The listing builds one solid part. Answer for the finished solid, in the listing's coordinates (mm). A direction names the side the tool comes from. Round coordinates to 2 decimals unless told otherwise and drop trailing zeros. Use a Markdown table: item, result. Add a question column.
Q1. Given pin 1 Ø6 at (x, y) = (-12.5, -16) entering from +Z; pin 2 Ø3 at (y, z) = (-13.5, 18) entering from +X; pin 3 Ø10 at (y, z) = (-21, -25) entering from +X, each flat-ended and moving along its own axis, determine where each tip first touches the part or whether it passes through.
Q2. Consider line 1 (Z direction, x = -29, y = -20.75); line 2 (Z direction, x = 29, y = -1.5); line 3 (Z direction, x = -17, y = -15). Determine where each line is inside the solid, lowest interval first.
Q3. For a pull along Z with two mould halves and no side action, classify faces 1 (the cylindrical face through (-3.974, -12.325, 33.948)), 2 (the cylindrical face through (-29.04, -12.32, 3.25)) as released by +Z, released by -Z, zero draft, split by the parting line, or undercut.
Q4. Which of the six approach directions +Z, -Z, +X, -X, +Y, -Y give full straight-line access (tool end or side, diameter ignored) to faces 3 (the cylindrical face through (-23.524, -12.325, 17.336)), 4 (the cylindrical face through (30.35, -12.32, 15.4)), 5 (the cylindrical face through (5.243, -12.325, -28.881)), 6 (the cylindrical face through (-17.336, -12.325, -23.524))?
from build123d import *

# Parameters (mm, degrees)
F1_DEPTH = 25
F2_COUNT = 12
F3_R     = 5.594929
F4_DEPTH = 45.5


with BuildPart() as f1:
    # F0 (on Front) → F1 (new body)
    with BuildSketch(Plane.XZ):
        with BuildLine():
            ThreePointArc((-5.207343, 26.350902), (-17.053073, -20.752811), (26.8605, 0))
            ThreePointArc((26.8605, 0), (20.131278, 17.782523), (3.315285, 26.655119))
            ThreePointArc((3.315285, 26.655119), (-0.958179, 26.843404), (-5.207343, 26.350902))
        make_face()
        with BuildLine():
            ThreePointArc((-5.207343, 26.350902), (-0.958179, 26.843404), (3.315285, 26.655119))
            ThreePointArc((3.315285, 26.655119), (3.247938, 29.073857), (2.798331, 31.451394))
            ThreePointArc((2.798331, 31.451394), (1.82091, 34.016407), (0.364343, 36.343005))
            ThreePointArc((0.364343, 36.343005), (-1.075338, 33.452857), (-2.616887, 36.289979))
            ThreePointArc((-2.616887, 36.289979), (-3.989795, 33.913056), (-4.875382, 31.314906))
            ThreePointArc((-4.875382, 31.314906), (-5.245453, 28.846552), (-5.207343, 26.350902))
        make_face()
    extrude(amount=F1_DEPTH)

    # F2: F1 ×12 about axis
    f2_axis = Axis((0, 0, 0), (0, 1, 0))


with BuildPart() as f1_1:
    add(f1.part)
    for i in range(1, F2_COUNT):
        add(f1.part.rotate(f2_axis, i * 360 / F2_COUNT))

    # F3 (on face) → F4 (cut)
    with BuildSketch(Plane.XZ.offset(25)):
        Circle(F3_R)
    extrude(amount=-F4_DEPTH, mode=Mode.SUBTRACT)


solid = f1_1.part
Checked values:
| question | item | result |
|---|---|---|
| 1 | pin 1 | stops at z = 30.41 |
| 1 | pin 2 | stops at x = 31.66 |
| 1 | pin 3 | stops at x = 20.48 |
| 2 | line 1 | z = -20.48 to -20.12, -17.07 to -13.68, -5.23 to 3.26, 10.94 to 18.61 |
| 2 | line 2 | z = -18.61 to -10.94, -3.26 to 5.23, 13.68 to 17.07, 20.12 to 20.48 |
| 2 | line 3 | z = -29.31 to -22.82, -20.8 to 29.12, 30.87 to 31.27 |
| 3 | face 1 | released by +Z |
| 3 | face 2 | undercut |
| 4 | face 3 | +Z, +Y, -Y |
| 4 | face 4 | +X, +Y, -Y |
| 4 | face 5 | +Y, -Y |
| 4 | face 6 | -X, +Y, -Y |
